Build history of the part. All positions in model axes, mm. A direction names the side the tool comes from. Give positions to 0.01 mm unless a question says otherwise; leave off trailing zeros. Write each loop counter-clockwise with the first axis right and the second up, starting at its lowest first coordinate (ties: lowest second). Pieces come first, ordered by that corner, then holes.
from build123d import *

# Parameters (mm, degrees)
SKETCH5_R          = 2
CUT_EXTRUDE2_DEPTH = 44.764369069
SKETCH6_R          = 4
CUT_EXTRUDE3_DEPTH = 22
SKETCH7_R          = 4.5
CUT_EXTRUDE4_DEPTH = 22
CUT_EXTRUDE5_DEPTH = 22
CUT_EXTRUDE6_DEPTH = 44.764369185


with BuildPart() as part:
    # Sketch2 → Revolve1 (revolve)
    with BuildSketch(Plane(origin=(0, 0, 0), x_dir=(0, 0, -1), z_dir=(1, 0, 0)), mode=Mode.PRIVATE) as revolve1_sk:
        Polygon((-18.45, 25), (-25.4, 4), (-25.4, 0), (-15, 0), (-15, 22), (0, 22), (0, 25), align=None)
    revolve(revolve1_sk.sketch.rotate(Axis((0, 0, 0), (0, 1, 0)), 180), axis=Axis((0, 0, 0), (0, 1, 0)))

    # Sketch5 → Cut-Extrude2 (cut, through all)
    with BuildSketch(Plane(origin=(0, 25, 0), x_dir=(1, 0, 0), z_dir=(0, 1, 0))):
        with Locations(Location((-15.556349186, -15.556349186, 0), (0, 0, 270))):
            Circle(SKETCH5_R)
        with Locations(Location((15.556349186, -15.556349186, 0), (0, 0, 270))):
            Circle(SKETCH5_R)
    extrude(amount=-CUT_EXTRUDE2_DEPTH, mode=Mode.SUBTRACT)

    # Sketch6 → Cut-Extrude3 (cut)
    with BuildSketch(Plane(origin=(0, 4, 0), x_dir=(-1, 0, 0), z_dir=(0, -1, 0))):
        with Locations((15.556349186, -15.556349186)):
            Circle(SKETCH6_R)
        with Locations((-15.556349186, -15.556349186)):
            Circle(SKETCH6_R)
    extrude(amount=-CUT_EXTRUDE3_DEPTH, mode=Mode.SUBTRACT)

    # Sketch7 → Cut-Extrude4 (cut)
    with BuildSketch(Plane(origin=(0, 0, 0), x_dir=(-1, 0, 0), z_dir=(0, -1, 0))):
        with Locations((15.556349186, 15.556349186)):
            Circle(SKETCH7_R)
        with Locations((-15.556349186, 15.556349186)):
            Circle(SKETCH7_R)
    extrude(amount=-CUT_EXTRUDE4_DEPTH, mode=Mode.SUBTRACT)

    # Sketch10 → Cut-Extrude5 (cut)
    with BuildSketch(Plane.XZ):
        with BuildLine():
            Line((-14.704067619, 2.964860106), (-16.680641023, -6.837851641))
            Line((-16.680641023, -6.837851641), (-20.322553732, -15.236594429))
            ThreePointArc((-20.322553732, -15.236594429), (-17.924840594, -17.996113183), (-15.155828757, -20.382856883))
            ThreePointArc((-15.155828757, -20.382856883), (0, -25.4), (15.155828757, -20.382856883))
            ThreePointArc((15.155828757, -20.382856883), (17.924840594, -17.996113183), (20.322553732, -15.236594429))
            Line((20.322553732, -15.236594429), (16.680641023, -6.837851641))
            Line((16.680641023, -6.837851641), (14.704067619, 2.964860106))
            ThreePointArc((14.704067619, 2.964860106), (0, 15), (-14.704067619, 2.964860106))
        make_face()
    extrude(amount=-CUT_EXTRUDE5_DEPTH, mode=Mode.SUBTRACT)

    # Sketch14 → Cut-Extrude6 (cut, through all)
    with BuildSketch(Plane(origin=(0, 25, 0), x_dir=(1, 0, 0), z_dir=(0, 1, 0))):
        with BuildLine():
            ThreePointArc((17.441336231, 8.592117572), (0, 19.442857143), (-17.441336231, 8.592117572))
            ThreePointArc((-17.441336231, 8.592117572), (0, 5.504168361), (17.441336231, 8.592117572))
        make_face()
    extrude(amount=-CUT_EXTRUDE6_DEPTH, mode=Mode.SUBTRACT)


solid = part.part
(1) Saw through at B-B, the plane z = 0. List the corners of the cut face in (x, y).
(2) Saw through at C-C, the plane y = 19.5. List the corners of the cut face in (x, z), plus the area to 3 significant figures.
(3) Drop flat-ended pins along their axis: pin 1 (5 mm diameter, centred on x = 15.56, z = 15.56, fed in from +Y); pin 2 (4 mm diameter, centred on y = 19.5, z = 20.5, fed in from +X); pin 3 (5 mm diameter, centred on y = 22, z = -6.5, fed in from +X); pin 4 (2.5 mm diameter, centred on x = -15.56, z = 15.56, fed in from +Y). Give the stop position or say it passes through.
(4) 3-axis set-ups, long thin cutter, end or side, ignore diameter. For faces 1 (the face through (14, 4, 14)), 2 (the face through (0, 11, 15)), 3 (the face through (-0.249, 23.521, -5.505)): which of +Z, -Z, +X, -X, +Y, -Y reach the whole face in a straight line?
(5) Saw through at A-A, the plane x = 0. List the corners of the cut face in (y, z), plus the area to 3 significant figures.
(6) Probe line 1 (X direction, y = 12.75, z = 12.5); line 2 (X direction, y = 8.25, z = -2); line 3 (Y direction, x = 7, z = -3). List the from-to ranges inside material, lowest first.
Computed values:
1. outline: (-25.4, 0) - (-15.3, 0) - (-15.3, 22) - (15.3, 22) - (15.3, 0) - (25.4, 0) - (25.4, 4) - (18.45, 25) - (-18.45, 25) - (-25.4, 4) - close
2. outline: (-17.87, -9.57) - (-16.68, -6.84) - (-14.7, 2.96) arc R15 cw to (14.7, 2.96) - (16.68, -6.84) - (17.87, -9.57) arc R20.27 ccw to (16.56, 11.69) arc R4 cw to (11.69, 16.56) arc R20.27 ccw to (-11.69, 16.56) arc R4 cw to (-16.56, 11.69) arc R20.27 ccw to start
2. area: 329 mm2
3. pin 1: stops at y = 4
3. pin 2: stops at x = 8.57
3. pin 3: stops at x = 19.47
3. pin 4: passes through
4. face 1: +Y
4. face 2: -Z, -Y
4. face 3: -Z, +Y, -Y
5. outline: (0, 15) - (22, 15) - (22, -5.5) - (25, -5.5) - (25, 18.45) - (4, 25.4) - (0, 25.4) - close
5. area: 249 mm2
6. line 1: x = -18.71 to -18.14, -12.98 to -8.29, 8.29 to 12.98, 18.14 to 18.71
6. line 2: x = -23.91 to -15.71, 15.71 to 23.91
6. line 3: y = 22 to 25
